Read the model definition and answer for the solid it produces. Units are mm, in the model's axes. Face numbers are marked on the shaded views. Coordinates: 2 decimals unless noted, no trailing zeros. Order: outer loops, then holes, each group sorted by start corner. A loop starts at its lowest first (then second) coordinate and runs counter-clockwise, first axis right, second up. Notation, with made-up numbers: M -21,38.25 L 29,38.25 A15 cw 29,61.25 Z; hole C 29.5,-1 d5. An arc over 180 degrees is marked long. Use a Markdown table: item, result. Add a question column.
1) Find section B-B on x = -18. Write down the section's boundary in (y, z).
2) The mould has two halves that part along X. Classify the marked faces 1, 2, 3 and 4: released by +X, released by -X, zero draft, split by the parting line, or undercut.
3) Find section A-A on z = 0. Write down the section's boundary in (x, y).
4) Each of these flat-tipped pins is pushed along its axis until it touches: pin 1 Ø3 at (x, y) = (-11, 3.5) entering from +Z; pin 2 Ø1 at (x, y) = (-30.5, 3) entering from -Z; pin 3 Ø3 at (x, y) = (-2, 2.5) entering from +Z; pin 4 Ø1 at (x, z) = (-25.5, 9) entering from -Y. Where does it stop, or does it pass through?
5) Find the intervals of material crossed by probe 1 along X at (y, z) = (1, -1); probe 2 along Z at (x, y) = (0.5, 3.5); probe 3 along Z at (x, y) = (-6, 6), in increasing order. Write a range as [from, to].
6) Find section C-C on z = 10. Write down the section's boundary in (x, y) (3 decimals).
from build123d import *

# Parameters (mm, degrees)
SKETCH1_R           = 2.4892
BOSS_EXTRUDE1_DEPTH = 6.35
FILLET1_R           = 2.54
FILLET2_R           = 2.54


with BuildPart() as part:
    # Sketch1 → Boss-Extrude1 (new body)
    with BuildSketch(Plane(origin=(0, 0, 0), x_dir=(1, 0, 0), z_dir=(0, 1, 0))):
        with BuildLine():
            Line((-1.600744285, 5.433302805), (-4.502878037, 4.373943057))
            Line((-4.502878037, 4.373943057), (-7.566118931, 1.089743665))
            Line((-7.566118931, 1.089743665), (-43.208775226, -11.210846355))
            Line((-43.208775226, -11.210846355), (-43.907997659, -11.677108885))
            Line((-43.907997659, -11.677108885), (0, -7.791786745))
            Line((0, -7.791786745), (0, -5.6642))
            ThreePointArc((0, -5.6642), (5.606178529, 0.808655641), (-1.600744285, 5.433302805))
        make_face()
        with Locations(Location((0, 0, 0), (0, 0, 270))):
            Circle(SKETCH1_R, mode=Mode.SUBTRACT)
    extrude(amount=BOSS_EXTRUDE1_DEPTH)

    # Fillet1
    # the kernel refuses this fillet: 2.54 mm, written as the material it adds along each edge
    with BuildSketch(Plane(origin=(-7.566118931, 0, -1.089743665), x_dir=(0.6820787973115132, 0, -0.7312786844001947), z_dir=(0, 1, 0))) as fillet1_piece_1:
        with BuildLine():
            CenterArc((FILLET1_R * 0.248898879334, FILLET1_R), FILLET1_R, 242.04630063, 27.95369937)
            Line((-FILLET1_R * 0.219859021674, FILLET1_R * 0.11667331624), (0, 0))
            Line((0, 0), (FILLET1_R * 0.248898879334, 0))
        make_face()
    extrude(amount=6.35)
    # the kernel refuses this fillet: 2.54 mm, written as the material it takes off along each edge
    with BuildSketch(Plane(origin=(0, -5.793464316, 7.791786745), x_dir=(0, 0, -1), z_dir=(0, 1, 0))) as fillet1_2_piece_1:
        with BuildLine():
            CenterArc((2.325851575, 2.532250196), FILLET1_R, 185.056806539, 80.466301584)
            Line((-0.204262229, 2.308365991), (0, 0))
            Line((0, 0), (2.127586745, 0))
        make_face()
    extrude(amount=17.936928632, mode=Mode.SUBTRACT)
    with BuildSketch(Plane(origin=(-1.600744285, -0.311653756, -5.433302805), x_dir=(-0.9393728970341759, 0, 0.34289730287306086), z_dir=(0, 1, 0))) as fillet1_2_piece_2:
        with BuildLine():
            CenterArc((0.092583262, 2.54), FILLET1_R, 265.101357171, 4.898642829)
            ThreePointArc((-0.124315777, 0.009277809), (-0.062183413, 0.004296891), (0, 0))
            Line((0, 0), (0.092583262, 0))
        make_face()
    extrude(amount=6.973307511, mode=Mode.SUBTRACT)
    with BuildSketch(Plane(origin=(-4.502878037, -1.520996143, -4.373943057), x_dir=(0.9393728970341768, 0, -0.34289730287305803), z_dir=(0, 1, 0))) as fillet1_2_piece_3:
        with BuildLine():
            CenterArc((FILLET1_R * 0.239526951609, -FILLET1_R), FILLET1_R, 90, 26.940206001)
            Line((-FILLET1_R * 0.213533444751, -FILLET1_R * 0.108520175635), (0, 0))
            Line((0, 0), (FILLET1_R * 0.239526951609, 0))
        make_face()
    extrude(amount=9.391992285, mode=Mode.SUBTRACT)

    # Fillet2
    fillet2_edges = [part.edges().sort_by_distance(p)[0] for p in [
        (0, 3.175, 5.6642),
    ]]
    fillet(fillet2_edges, radius=FILLET2_R)


solid = part.part
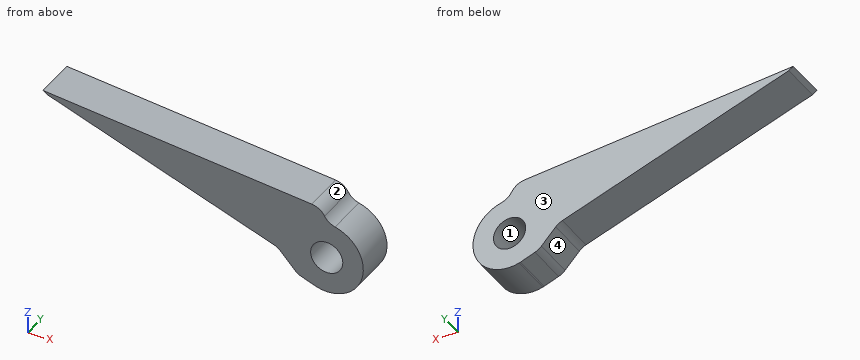
Check result:
| question | item | result |
|---|---|---|
| 1 | outline | M 0,2.51 L 6.35,2.51 L 6.35,9.38 L 0,9.38 Z |
| 2 | face 1 | undercut |
| 2 | face 2 | released by +X |
| 2 | face 3 | zero draft |
| 2 | face 4 | released by -X |
| 3 | outline | M -10.72,0 L -2.49,0 L -2.49,6.35 L -10.72,6.35 Z; M 2.49,0 L 5.66,0 L 5.66,6.35 L 2.49,6.35 Z |
| 4 | pin 1 | stops at z = 8.9 |
| 4 | pin 2 | stops at z = 6.65 |
| 4 | pin 3 | stops at z = 8.1 |
| 4 | pin 4 | stops at y = 0 |
| 5 | probe 1 | x = [-7.88, -2.28], [2.28, 5.58] |
| 5 | probe 2 | z = [-5.64, -2.44], [2.44, 5.85] |
| 5 | probe 3 | z = [-2.77, 8.32] |
| 6 | outline | M -39.7,0 L -24.955,0 L -24.955,6.35 L -39.7,6.35 Z |
